from build123d import *

# Parameters (mm, degrees)
SKETCH_1_W           = 30
SKETCH_1_H           = 28
EXTRUDE_1_DEPTH      = 10
CUT_EXTRUDE_2_DEPTH  = 0.8
M1_4X0_3_2_D         = 1.1
M1_4X0_3_2_DEPTH     = 3.7
M1_4X0_3_2_TIP       = 0.33047334
CUT_EXTRUDE_3_DEPTH  = 4
CUT_EXTRUDE_4_DEPTH  = 0.5
SKETCH_12_W          = 30
SKETCH_12_H          = 4.25
CUT_EXTRUDE_5_DEPTH  = 10
SKETCH_14_W          = 23
SKETCH_14_H          = 23.75
CUT_EXTRUDE_7_DEPTH  = 5
SKETCH_23_W          = 4
SKETCH_23_H          = 23.75
EXTRUDE_4_DEPTH      = 9.1
SKETCH_24_W          = 30
SKETCH_24_H          = 7.75
CUT_EXTRUDE_8_DEPTH  = 20
SKETCH_25_W          = 7
SKETCH_25_H          = 16
EXTRUDE_5_DEPTH      = 4.1
SKETCH_26_W          = 3
SKETCH_26_H          = 0.8
CUT_EXTRUDE_9_DEPTH  = 4.1
SKETCH_28_W          = 1.1
SKETCH_28_H          = 3
CUT_EXTRUDE_11_DEPTH = 4
CUT_EXTRUDE_START    = -4
SKETCH_29_R          = 0.1
CUT_EXTRUDE_12_DEPTH = 4


with BuildPart() as part:
    # 草图1 → 凸台-拉伸1 (new body)
    with BuildSketch(Plane.XY):
        with Locations((7.449728974, 2.736434109)):
            Rectangle(SKETCH_1_W, SKETCH_1_H)
    extrude(amount=EXTRUDE_1_DEPTH)

    # 草图2 → 切除-拉伸2 (cut)
    with BuildSketch(Plane(origin=(0, 0, 0), x_dir=(-1, 0, 0), z_dir=(0, 0, -1))):
        with BuildLine():
            Line((5.050271026, 16.736434109), (-15.449728974, 16.736434109))
            Line((-15.449728974, 16.736434109), (-15.449728974, 3.736434109))
            ThreePointArc((-15.449728974, 3.736434109), (-14.571049317, 1.615113765), (-12.449728974, 0.736434109))
            Line((-12.449728974, 0.736434109), (2.050271026, 0.736434109))
            ThreePointArc((2.050271026, 0.736434109), (4.17159137, 1.615113765), (5.050271026, 3.736434109))
            Line((5.050271026, 3.736434109), (5.050271026, 16.736434109))
        make_face()
    extrude(amount=-CUT_EXTRUDE_2_DEPTH, mode=Mode.SUBTRACT)

    # M1.4x0.3 螺纹孔2
    with Locations(Plane(origin=(0, 0, 0.8), x_dir=(-1, 0, 0), z_dir=(0, 0, -1))):
        with Locations((-12.199728974, 8.736434109), (1.800271026, 8.736434109)):
            Hole(M1_4X0_3_2_D / 2, depth=M1_4X0_3_2_DEPTH)
            with Locations((0, 0, -(M1_4X0_3_2_DEPTH + M1_4X0_3_2_TIP / 2))):  # 118° drill point
                Cone(0, M1_4X0_3_2_D / 2, M1_4X0_3_2_TIP, mode=Mode.SUBTRACT)

    # 草图10 → 切除-拉伸3 (cut)
    with BuildSketch(Plane(origin=(0, 16.736434109, 0), x_dir=(1, 0, 0), z_dir=(0, 1, 0))):
        with BuildLine():
            Line((9.249728974, -0.8), (8.149728974, -0.8))
            Line((8.149728974, -0.8), (8.149728974, -3.7))
            ThreePointArc((8.149728974, -3.7), (8.07901805, -3.870710433), (8.249728974, -3.800000693))
            Line((8.249728974, -3.800000693), (9.14947862, -3.800000693))
            ThreePointArc((9.14947862, -3.800000693), (9.320100726, -3.870799843), (9.249728974, -3.700001016))
            Line((9.249728974, -3.700001016), (9.249728974, -0.8))
        make_face()
        with BuildLine():
            Line((1.149728974, -0.8), (2.249728974, -0.8))
            Line((2.249728974, -0.8), (2.249728974, -3.696415438))
            ThreePointArc((2.249728974, -3.696415438), (2.32297432, -3.873245346), (2.146144411, -3.8))
            Line((2.146144411, -3.8), (1.245429293, -3.8))
            ThreePointArc((1.245429293, -3.8), (1.082058629, -3.867670345), (1.149728974, -3.704299681))
            Line((1.149728974, -3.704299681), (1.149728974, -0.8))
        make_face()
    extrude(amount=-CUT_EXTRUDE_3_DEPTH, mode=Mode.SUBTRACT)

    # 草图11 → 切除-拉伸4 (cut)
    with BuildSketch(Plane(origin=(0, 0, 0), x_dir=(-1, 0, 0), z_dir=(0, 0, -1))):
        with BuildLine():
            Line((-7.549728974, -2.063565891), (-2.849728974, -2.063565891))
            ThreePointArc((-2.849728974, -2.063565891), (-2.422952278, -2.240342587), (-2.599728974, -1.813565891))
            Line((-2.599728974, -1.813565891), (-2.599728974, 0.736434109))
            Line((-2.599728974, 0.736434109), (-7.799728974, 0.736434109))
            Line((-7.799728974, 0.736434109), (-7.799728974, -1.813565891))
            ThreePointArc((-7.799728974, -1.813565891), (-7.976505669, -2.240342587), (-7.549728974, -2.063565891))
        make_face()
    extrude(amount=-CUT_EXTRUDE_4_DEPTH, mode=Mode.SUBTRACT)

    # 草图12 → 切除-拉伸5 (cut)
    with BuildSketch(Plane(origin=(0, 0, 0), x_dir=(-1, 0, 0), z_dir=(0, 0, -1))):
        with Locations((-7.449728974, -9.138565891)):
            Rectangle(SKETCH_12_W, SKETCH_12_H)
    extrude(amount=-CUT_EXTRUDE_5_DEPTH, mode=Mode.SUBTRACT)

    # 草图14 → 切除-拉伸7 (cut)
    with BuildSketch(Plane.XY.offset(10)):
        with Locations((3.949728974, 4.861434109)):
            Rectangle(SKETCH_14_W, SKETCH_14_H)
    extrude(amount=-CUT_EXTRUDE_7_DEPTH, mode=Mode.SUBTRACT)

    # 草图23 → 凸台-拉伸4 (add)
    with BuildSketch(Plane.XY.offset(5)):
        with Locations((-5.550271026, 4.861434109)):
            Rectangle(SKETCH_23_W, SKETCH_23_H)
    extrude(amount=EXTRUDE_4_DEPTH)

    # 草图24 → 切除-拉伸8 (cut)
    with BuildSketch(Plane(origin=(0, 0, 0), x_dir=(-1, 0, 0), z_dir=(0, 0, -1))):
        with Locations((-7.449728974, -3.138565891)):
            Rectangle(SKETCH_24_W, SKETCH_24_H)
    extrude(amount=-CUT_EXTRUDE_8_DEPTH, mode=Mode.SUBTRACT)

    # 草图25 → 凸台-拉伸5 (add)
    with BuildSketch(Plane.XY.offset(10)):
        with Locations((18.949728974, 8.736434109)):
            Rectangle(SKETCH_25_W, SKETCH_25_H)
    extrude(amount=EXTRUDE_5_DEPTH)

    # 草图26 → 切除-拉伸9 (cut)
    with BuildSketch(Plane.XZ.offset(-0.736434109)):
        with Locations((13.949728974, 0.4)):
            Rectangle(SKETCH_26_W, SKETCH_26_H)
        with Locations((-3.550271026, 0.4)):
            Rectangle(SKETCH_26_W, SKETCH_26_H)
    extrude(amount=-CUT_EXTRUDE_9_DEPTH, mode=Mode.SUBTRACT)

    # 草图28 → 切除-拉伸11 (cut)
    with BuildSketch(Plane.XZ.offset(-0.736434109)):
        with Locations((8.699728974, 2.3)):
            Rectangle(SKETCH_28_W, SKETCH_28_H)
        with Locations((1.699728974, 2.3)):
            Rectangle(SKETCH_28_W, SKETCH_28_H)
    extrude(amount=-CUT_EXTRUDE_11_DEPTH, mode=Mode.SUBTRACT)

    # 草图29 → 切除-拉伸12 (cut)
    with BuildSketch(Plane.XZ.offset(-0.736434109).offset(CUT_EXTRUDE_START)):
        with Locations((9.249728974, 3.8)):
            Circle(SKETCH_29_R)
        with Locations((8.149728974, 3.8)):
            Circle(SKETCH_29_R)
        with Locations((2.249728974, 3.8)):
            Circle(SKETCH_29_R)
        with Locations((1.149728974, 3.8)):
            Circle(SKETCH_29_R)
    extrude(amount=CUT_EXTRUDE_12_DEPTH, mode=Mode.SUBTRACT)


solid = part.part
Check sheet for the modelled part. Datum: model origin and axes. Units: mm. A direction names the side the tool comes from. Round coordinates to 2 decimals unless told otherwise and drop trailing zeros. Order: outer loops, then holes, each group sorted by start corner. A loop starts at its lowest first (then second) coordinate and runs counter-clockwise, first axis right, second up. Notation, with made-up numbers: M 74.25,-22.5 L 97.25,-22.5 A8 cw 97.25,-16.5 Z; hole C -15.5,-34 d11. An arc over 180 degrees is marked long. One line per item, written item: value. Start each with the question number.
1. Access from +Z, -Z, +X, -X, +Y, -Y to the whole of each face (thin tool, end or side, straight path). Record for faces 4 (the flat face through (1.15, 3, 2)), 5 (the flat face through (5, 9, 0.8)), 6 (the flat face through (1.7, 14.8, 3.8)), 7 (the flat face through (6, 9, 5)).
2. Section check A-A on z = 8.5. Enter the section's corners in (x, y), and give its area (3 significant figures).
3. Gauge pin test, flat ends, axial feed: P1, Ø8, axis at x = 5, y = 8, coming from the -Z side; P2, Ø0.9, axis at x = -1.8, y = 8.74, coming from the +Z side; P3, Ø0.6, axis at x = 8.5, z = 2.5, coming from the +Y side; P4, Ø8, axis at x = 16.5, y = 11, coming from the -Z side. Record the tip position at first contact, or that the pin passes through.
4. Section check D-D on y = 15.25. Enter the section's corners in (x, z).
5. Section check C-C on x = 14. Enter the section's corners in (y, z).
6. Release check for a two-part mould opening along X. For faces 1 (the flat face through (19, 9, 14.1)), 2 (the flat face through (-7.55, 9, 7)), 3 (the flat face through (-3.55, 9, 9)) record: released by +X, released by -X, zero draft, split by the parting line, or undercut.
7. Scan lines: line 1 along X through (y, z) = (14.25, 6); line 2 along Z through (x, y) = (-5, 15); line 3 along Z through (x, y) = (13.75, 7.75). Record each from-to range of solid material in increasing order.
8. Section check B-B on y = 5.75. Enter the section's corners in (x, z), and give its area (3 significant figures).
Results found:
1. face 4: -Z, -Y
1. face 5: -Z, +Y, -Y
1. face 6: -Z, +Y
1. face 7: +Z, +Y, -Y
2. outline: M -7.55,0.74 L -3.55,0.74 L -3.55,16.74 L -7.55,16.74 Z; M 15.45,0.74 L 22.45,0.74 L 22.45,16.74 L 15.45,16.74 Z
2. area: 176 mm^2
3. P1: z = 0.8
3. P2: z = 5
3. P3: y = 12.74
3. P4: z = 0
4. outline: M -7.55,0 L -5.05,0 L -5.05,0.8 L 1.15,0.8 L 1.15,3.7 A0.1 cw long 1.25,3.8 L 2.15,3.8 A0.1 cw long 2.25,3.7 L 2.25,0.8 L 8.15,0.8 L 8.15,3.7 A0.1 cw long 8.25,3.8 L 9.15,3.8 A0.1 cw long 9.25,3.7 L 9.25,0.8 L 15.45,0.8 L 15.45,0 L 22.45,0 L 22.45,14.1 L 15.45,14.1 L 15.45,5 L -3.55,5 L -3.55,14.1 L -7.55,14.1 Z
5. outline: M 0.74,0.8 L 16.74,0.8 L 16.74,5 L 0.74,5 Z
6. face 1: zero draft
6. face 2: released by -X
6. face 3: undercut
7. line 1: -7.55 to -3.55, 15.45 to 22.45
7. line 2: 0.8 to 14.1
7. line 3: 0.8 to 5
8. outline: M -7.55,0 L -5.05,0 L -5.05,0.8 L 15.45,0.8 L 15.45,0 L 22.45,0 L 22.45,14.1 L 15.45,14.1 L 15.45,5 L -3.55,5 L -3.55,14.1 L -7.55,14.1 Z
8. area: 234 mm^2
